from build123d import *

# Parameters (mm, degrees)
BOSS_EXTRUDE1_DEPTH = 2
SKETCH5_R           = 5
CUT_EXTRUDE1_DEPTH  = 28


with BuildPart() as part:
    # Sketch2 → Boss-Extrude1 (new body)
    with BuildSketch(Plane.XY):
        with BuildLine():
            Line((-20.5, -1), (-13.5, -1))
            ThreePointArc((-13.5, -1), (-12.085786438, -0.414213562), (-11.5, 1))
            Line((-11.5, 1), (-11.5, 7))
            ThreePointArc((-11.5, 7), (-11, 7.5), (-10.5, 7))
            Line((-10.5, 7), (-10.5, 0))
            Line((-10.5, 0), (-10.5, -7))
            ThreePointArc((-10.5, -7), (-8, -9.5), (-5.5, -7))
            Line((-5.5, -7), (-5.5, 0))
            Line((-5.5, 0), (-5.5, 7))
            ThreePointArc((-5.5, 7), (-5, 7.5), (-4.5, 7))
            Line((-4.5, 7), (-4.5, 0))
            Line((-4.5, 0), (-4.5, -7))
            ThreePointArc((-4.5, -7), (-2, -9.5), (0.5, -7))
            Line((0.5, -7), (0.5, 0))
            Line((0.5, 0), (0.5, 7))
            ThreePointArc((0.5, 7), (1, 7.5), (1.5, 7))
            Line((1.5, 7), (1.5, 0))
            Line((1.5, 0), (1.5, -7))
            ThreePointArc((1.5, -7), (4, -9.5), (6.5, -7))
            Line((6.5, -7), (6.5, -1))
            Line((6.5, -1), (13.5, -1))
            ThreePointArc((13.5, -1), (14.5, 0), (13.5, 1))
            Line((13.5, 1), (6.5, 1))
            ThreePointArc((6.5, 1), (5.085786438, 0.414213562), (4.5, -1))
            Line((4.5, -1), (4.5, -7))
            ThreePointArc((4.5, -7), (4, -7.5), (3.5, -7))
            Line((3.5, -7), (3.5, 0))
            Line((3.5, 0), (3.5, 7))
            ThreePointArc((3.5, 7), (1, 9.5), (-1.5, 7))
            Line((-1.5, 7), (-1.5, 0))
            Line((-1.5, 0), (-1.5, -7))
            ThreePointArc((-1.5, -7), (-2, -7.5), (-2.5, -7))
            Line((-2.5, -7), (-2.5, 0))
            Line((-2.5, 0), (-2.5, 7))
            ThreePointArc((-2.5, 7), (-5, 9.5), (-7.5, 7))
            Line((-7.5, 7), (-7.5, 0))
            Line((-7.5, 0), (-7.5, -7))
            ThreePointArc((-7.5, -7), (-8, -7.5), (-8.5, -7))
            Line((-8.5, -7), (-8.5, 0))
            Line((-8.5, 0), (-8.5, 7))
            ThreePointArc((-8.5, 7), (-11, 9.5), (-13.5, 7))
            Line((-13.5, 7), (-13.5, 1))
            Line((-13.5, 1), (-20.5, 1))
            ThreePointArc((-20.5, 1), (-21.5, 0), (-20.5, -1))
        make_face()
    extrude(amount=BOSS_EXTRUDE1_DEPTH)

    # Sketch3 → Revolve1 (revolve)
    with BuildSketch(Plane(origin=(0, 0, 0), x_dir=(1, 0, 0), z_dir=(0, 1, 0)), mode=Mode.PRIVATE) as revolve1_sk:
        Polygon((-20.5, -2), (-25.5, -2), (-26.5, 2), (-26.5, 28), (-20.5, 28), align=None)
    revolve(revolve1_sk.sketch.rotate(Axis((-20.5, 0, 2), (0, 0, -1)), 168.463040967), axis=Axis((-20.5, 0, 2), (0, 0, -1)))

    # Sketch4 → Revolve2 (revolve)
    with BuildSketch(Plane(origin=(0, 0, 0), x_dir=(1, 0, 0), z_dir=(0, 1, 0)), mode=Mode.PRIVATE) as revolve2_sk:
        Polygon((13.5, -2), (18.5, -2), (19.5, 2), (19.5, 28), (13.5, 28), align=None)
    revolve(revolve2_sk.sketch.rotate(Axis((13.5, 0, 2), (0, 0, -1)), 169.524319524), axis=Axis((13.5, 0, 2), (0, 0, -1)))

    # Sketch5 → Cut-Extrude1 (cut)
    with BuildSketch(Plane(origin=(0, 0, -28), x_dir=(-1, 0, 0), z_dir=(0, 0, -1))):
        with Locations((-13.5, 0)):
            Circle(SKETCH5_R)
        with Locations((20.5, 0)):
            Circle(SKETCH5_R)
    extrude(amount=-CUT_EXTRUDE1_DEPTH, mode=Mode.SUBTRACT)


solid = part.part
The model under review builds one solid part; all positions refer to its coordinate system, in mm. A direction names the side the tool comes from. Round coordinates to 2 decimals unless told otherwise and drop trailing zeros. Order: outer loops, then holes, each group sorted by start corner. A loop starts at its lowest first (then second) coordinate and runs counter-clockwise, first axis right, second up. Notation, with made-up numbers: (-5, -1) -> (16, -1) arc R17 ccw to (16, 18) -> close; hole circle Ø10 at (42.5, -35.75). An arc over 180 degrees is marked (long way). Write item = value, one per line. Start each with the question number.
Item 1: Mouldability with a two-part tool opening along Y and no side actions: class faces 1 (the face through (14, 0, 0)), 2 (the face through (-8.1, -9.5, 1)), 3 (the face through (-2, -7.5, 1)) as released by +Y, released by -Y, zero draft, split by the parting line, or undercut.
Item 2: Consider section C-C on y = -0.5. Count the separate pieces of the cut face and the enclosed holes in it, plus the area to 3 significant figures.
Item 3: Consider section D-D on z = -0.5. Write out the cut boundary in (x, y) (3 decimals).
Item 4: For faces 4 (the face through (-11.5, 4, 1)), 5 (the face through (-14, 1, 1)), 6 (the face through (-20, 0, 0)), list the 3-axis set-ups (+Z, -Z, +X, -X, +Y, -Y) from which the entire face can be reached by the end or side of a thin tool; tool diameter is ignored.
Item 5: Consider section B-B on x = 13.5. Write out the cut boundary in (y, z), plus the area to 3 significant figures.
Item 6: Consider section A-A on z = -25. Write out the cut boundary in (x, y), plus the area to 3 significant figures.
Item 7: For line 1 along X through (y, z) = (0.5, -12); line 2 along Y through (x, z) = (13.5, -12.25); line 3 along X through (y, z) = (-3.5, -5), list the stretches that pass through material, from the lowest coordinate up.
Item 8: Clearance check with flat-ended pins moving along their axes: pin 1 Ø2 at (y, z) = (3, 1.5) entering from -X; pin 2 Ø2 at (y, z) = (-4, 1.5) entering from +X; pin 3 Ø1.6 at (y, z) = (-0.5, 1) entering from -X. State where each tip first meets the part, or that it passes through.
Conclusion:
q1.face_1 = undercut
q1.face_2 = released by -Y
q1.face_3 = released by +Y
q2.separate_pieces = 7
q2.enclosed_holes = 0
q2.area = 186 mm2
q3.outline = circle Ø11.25 at (-20.5, 0); circle Ø11.25 at (13.5, 0); hole circle Ø10 at (-20.5, 0); hole circle Ø10 at (13.5, 0)
q4.face_4 = +Z, -Z, -Y
q4.face_5 = +Z, +Y
q4.face_6 = -Z
q5.outline = (-6, -28) -> (-5, -28) -> (-5, 0) -> (5, 0) -> (5, -28) -> (6, -28) -> (6, -2) -> (5, 2) -> (-5, 2) -> (-6, -2) -> close
q5.area = 76.0 mm2
q6.outline = circle Ø12 at (-20.5, 0); circle Ø12 at (13.5, 0); hole circle Ø10 at (-20.5, 0); hole circle Ø10 at (13.5, 0)
q6.area = 69.1 mm2
q7.line_1 = -26.48 to -25.47, -15.53 to -14.52, 7.52 to 8.53, 18.47 to 19.48
q7.line_2 = -6 to -5, 5 to 6
q7.line_3 = -25.37 to -24.07, -16.93 to -15.63, 8.63 to 9.93, 17.07 to 18.37
q8.pin_1 = -25.3
q8.pin_2 = 17.72
q8.pin_3 = -25.94
